```python
from build123d import *

# Parameters (mm, degrees)
F1_DEPTH = 56
F3_DEPTH = 116
F5_D     = 12
F5_DEPTH = 5
F5_TIP   = 3.6051637142


# Not quite as in the source:
# - a feature names something its author has since deleted; it is built from what else it names


with BuildPart() as f1:
    # F0 (on Front) → F1 (new body)
    with BuildSketch(Plane.XZ):
        Polygon((1.5, 0), (2, 2), (12, 2), (12.5, 0), (58, 0), (58, 20), (-58, 20), (-58, 0), (-12.5, 0), (-12, 2), (-2, 2), (-1.5, 0), (0, 0), align=None)
    extrude(amount=F1_DEPTH)

    # F2 (on face) → F3 (cut, through all)
    with BuildSketch(Plane(origin=(-58, 0, 0), x_dir=(0, -1, 0), z_dir=(-1, 0, 0))):
        Polygon((28, 20), (20.0020753821, 20), (13, 10), (28, 10), align=None)
        Polygon((35.9979246179, 20), (28, 20), (28, 10), (43, 10), align=None)
    extrude(amount=-F3_DEPTH, mode=Mode.SUBTRACT)

    # F5
    with Locations(Plane.XY.offset(10)):
        with Locations((-1.5, -28)):
            Hole(F5_D / 2, depth=F5_DEPTH)
            with Locations((0, 0, -(F5_DEPTH + F5_TIP / 2))):  # 118° drill point
                Cone(0, F5_D / 2, F5_TIP, mode=Mode.SUBTRACT)


solid = f1.part
```
The listing builds one solid part. Answer for the finished solid, in the listing's coordinates (mm). A direction names the side the tool comes from. Give positions to 0.01 mm unless a question says otherwise; leave off trailing zeros. Order: outer loops, then holes, each group sorted by start corner. A loop starts at its lowest first (then second) coordinate and runs counter-clockwise, first axis right, second up. Notation, with made-up numbers: (89, 67.5) - (105, 67.5) arc R32 cw to (105, 98.5) - close; hole circle Ø9 at (36, 68.25). An arc over 180 degrees is marked (long way). Answer in a Markdown table with one row per item. Add a question column.
Q1. Which of the six approach directions +Z, -Z, +X, -X, +Y, -Y give full straight-line access (tool end or side, diameter ignored) to faces 1 (the cylindrical face through (-0.199, -33.857, 7.465)), 2 (the flat face through (-1, 0, 10)), 3 (the flat face through (-12.254, -27.608, 0.986)), 4 (the flat face through (-0.81, -16.55, 15.07)), 5 (the flat face through (1, -10, 20))?
Q2. The part is cut by section A-A (z = 18.75). Determine the outline of the cut face in (x, y), then the cut area to 3 significant figures.
Q3. Given P1, Ø8, axis at x = -6.5, y = -39, coming from the -Z side, flat-ended and moving along its own axis, determine where the tip first touches the part or whether it passes through.
Q4. The part is cut by section C-C (y = -52). Determine the outline of the cut face in (x, z), then the cut area to 3 significant figures.
Q5. The part is cut by section B-B (x = 23). Determine the outline of the cut face in (y, z).
Q6. For a pull along X with two mould halves and no side action, classify faces 6 (the flat face through (-58, -28, 8)), 7 (the flat face through (-36, -28, 0)), 8 (the flat face through (58, -28, 8)), 9 (the conical face through (-1.02, -28.92, 2.02)) as released by +X, released by -X, zero draft, split by the parting line, or undercut.
Q7. Find the intervals of material crossed by line 1 along Y through (x, z) = (-1.5, 7.4); line 2 along X through (y, z) = (-28, 6.8); line 3 along Z through (x, y) = (-33, -27), in increasing order. Write a range as [from, to].
Q8. The part is cut by section D-D (z = 13). Determine the outline of the cut face in (x, y).
Determined:
| question | item | result |
|---|---|---|
| 1 | face 1 | +Z |
| 1 | face 2 | +Z, -Z, +X, -X, +Y |
| 1 | face 3 | -Z, +Y, -Y |
| 1 | face 4 | +X, -X |
| 1 | face 5 | +Z, +X, -X, +Y, -Y |
| 2 | outline | (-58, -56) - (58, -56) - (58, -36.87) - (-58, -36.87) - close; (-58, -19.13) - (58, -19.13) - (58, 0) - (-58, 0) - close |
| 2 | area | 4,440 mm² |
| 3 | P1 | stops at z = 2 |
| 4 | outline | (-58, 0) - (-12.5, 0) - (-12, 2) - (-2, 2) - (-1.5, 0) - (1.5, 0) - (2, 2) - (12, 2) - (12.5, 0) - (58, 0) - (58, 20) - (-58, 20) - close |
| 4 | area | 2,280 mm² |
| 5 | outline | (-56, 0) - (0, 0) - (0, 20) - (-20, 20) - (-13, 10) - (-43, 10) - (-36, 20) - (-56, 20) - close |
| 6 | face 6 | released by -X |
| 6 | face 7 | zero draft |
| 6 | face 8 | released by +X |
| 6 | face 9 | undercut |
| 7 | line 1 | y = [-56, -34], [-22, 0] |
| 7 | line 2 | x = [-58, -7.5], [4.5, 58] |
| 7 | line 3 | z = [0, 10] |
| 8 | outline | (-58, -56) - (58, -56) - (58, -40.9) - (-58, -40.9) - close; (-58, -15.1) - (58, -15.1) - (58, 0) - (-58, 0) - close |
